```python
from build123d import *

# Parameters (mm, degrees)
F0_R     = 4
F1_DEPTH = 35
F2_R     = 5
F2_R_2   = 4
F3_DEPTH = 5
F4_R     = 3


with BuildPart() as f1:
    # F0 (on Front) → F1 (new body, symmetric)
    with BuildSketch(Plane.XZ):
        Circle(F0_R)
    extrude(amount=F1_DEPTH, both=True)

    # F2 (on face) → F3 (join)
    with BuildSketch(Plane.XZ.offset(35)):
        Circle(F2_R)
        Circle(F2_R_2, mode=Mode.SUBTRACT)
        Circle(F2_R_2)
    extrude(amount=F3_DEPTH)

    # F4
    f4_edges = [f1.edges().sort_by_distance(p)[0] for p in [
        (-5, -40, 0),
    ]]
    fillet(f4_edges, radius=F4_R)


solid = f1.part
```
Verification items for the finished model (mm, model axes). A direction names the side the tool comes from. Coordinates: 2 decimals unless noted, no trailing zeros. Loops run counter-clockwise (first coordinate to the right, second up) from the corner with the lowest first, then second, coordinate; pieces in that order, holes last. Notation, with made-up numbers: (-0.5, 6) -> (50.5, 6) arc R20 ccw to (50.5, 13) -> close; hole circle Ø11 at (87, -32). An arc over 180 degrees is marked (long way). Answer in a Markdown table with one row per item. Add a question column.
1. Access from +Z, -Z, +X, -X, +Y, -Y to the whole of each face (thin tool, end or side, straight path). Record for faces 1 (the face through (-0.867, -0.49, -3.905)), 2 (the face through (0, 35, 0)).
2. Material ranges on probe 1 along Z at (x, y) = (0, -11); probe 2 along X at (y, z) = (-16, 0.25); probe 3 along Y at (x, z) = (-3, -1), recorded low to high. Write a range as [from, to].
3. Depth check by flat-ended pin: P1, Ø1, axis at y = -17, z = 0.5, coming from the +X side; P2, Ø3, axis at y = -13.5, z = -3, coming from the -X side; P3, Ø3, axis at x = -2, y = -29.5, coming from the -Z side. Enter the tip coordinate at first touch or a pass-through.
4. Section check A-A, the plane y = -11. Enter the section's corners in (x, z), then the cut area to 3 significant figures.
Derived:
| question | item | result |
|---|---|---|
| 1 | face 1 | +Y |
| 1 | face 2 | +Z, -Z, +X, -X, +Y |
| 2 | probe 1 | z = [-4, 4] |
| 2 | probe 2 | x = [-3.99, 3.99] |
| 2 | probe 3 | y = [-39.77, 35] |
| 3 | P1 | stops at x = 4 |
| 3 | P2 | stops at x = -3.71 |
| 3 | P3 | stops at z = -3.97 |
| 4 | outline | circle Ø8 at (0, 0) |
| 4 | area | 50.3 mm² |
